Design review of the part shown in the three views and the two pictorial views. Dimensions are in mm from the part's minimum x, y and z. A direction names the side the tool comes from. Give positions to 0.01 mm unless a question says otherwise; leave off trailing zeros. Loops run counter-clockwise (first coordinate to the right, second up) from the corner with the lowest first, then second, coordinate; pieces in that order, holes last. Notation, with made-up numbers: (35.25, 33.5) - (73.25, 33.5) arc R35 ccw to (73.25, 68.5) - close; hole circle Ø10 at (6, 25). An arc over 180 degrees is marked (long way). Answer as a JSON object with one key per item and string values.
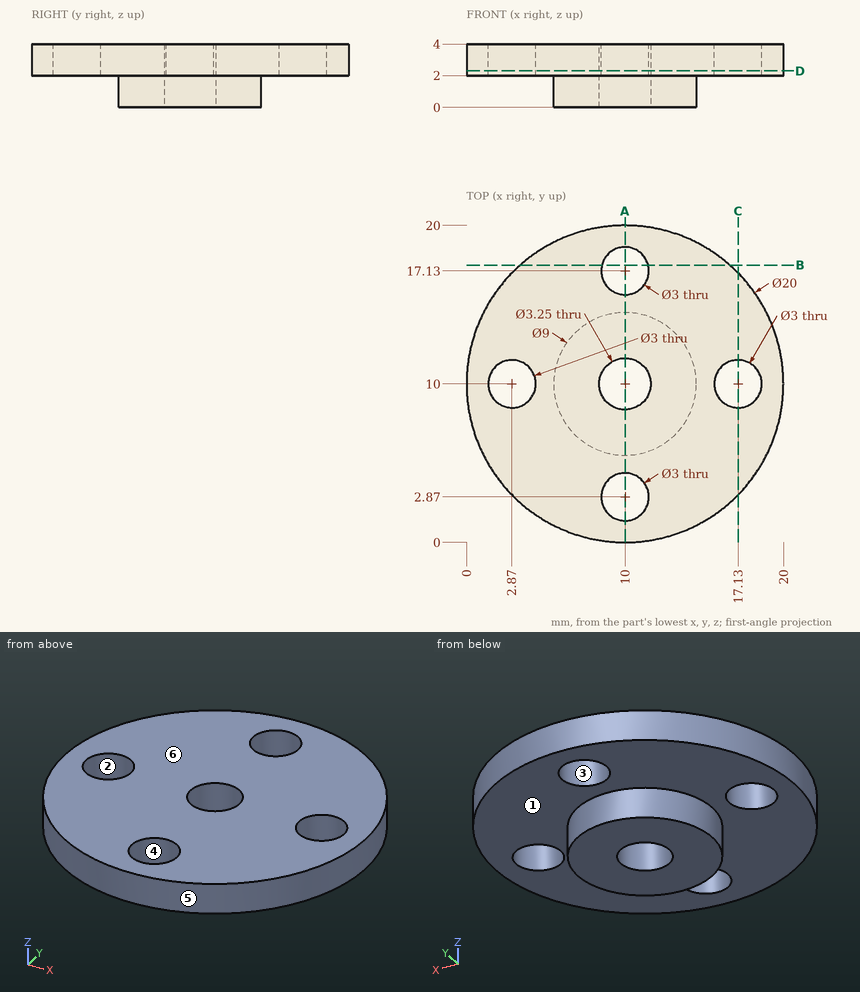
Q1. Clearance check with flat-ended pins moving along their axes: pin 1 Ø4 at (x, y) = (10, 10) entering from +Z; pin 2 Ø3.5 at (x, y) = (10, 2.87) entering from -Z. State where each tip first meets the part, or that it passes through.
Results:
{"pin 1": "stops at z = 4", "pin 2": "stops at z = 2"}
Q2. The part is to be moulded in two halves that separate along X. For the marked faces 3, 4, 5 and 6, say which applies: +X half, -X half, draft (parallel to the pull), parting line (faces both ways), or undercut.
Results:
{"face 3": "undercut", "face 4": "undercut", "face 5": "parting line", "face 6": "draft"}
Q3. Consider section D-D, the plane z = 2.3. State the section outline as (x, y) points (3 decimals).
Results:
{"outline": "circle Ø20 at (10, 10); hole circle Ø3 at (2.87, 10); hole circle Ø3.25 at (10, 10); hole circle Ø3 at (10, 2.87); hole circle Ø3 at (10, 17.13); hole circle Ø3 at (17.13, 10)"}
Q4. For the marked faces 1 and 2, list the 3-axis set-ups (+Z, -Z, +X, -X, +Y, -Y) from which the entire face can be reached by the end or side of a thin tool; tool diameter is ignored.
Results:
{"face 1": "-Z", "face 2": "+Z, -Z"}
Q5. To check wall thickness, follow probe 1 along Y at (x, z) = (10, 3.5) (3 decimals); probe 2 along Y at (x, z) = (9.5, 2.95); probe 3 along Z at (x, y) = (11.75, 18.5). State the ranges of each line that lie inside material, in increasing order. Write a range as [from, to].
Results:
{"probe 1": "y = [0, 1.37], [4.37, 8.375], [11.625, 15.63], [18.63, 20]", "probe 2": "y = [0.01, 1.46], [4.28, 8.45], [11.55, 15.72], [18.54, 19.99]", "probe 3": "z = [2, 4]"}
Q6. Consider section C-C, the plane x = 17.13. State the section outline as (y, z) points, plus the area to 3 significant figures.
Results:
{"outline": "(2.99, 2) - (8.5, 2) - (8.5, 4) - (2.99, 4) - close; (11.5, 2) - (17.01, 2) - (17.01, 4) - (11.5, 4) - close", "area": "22.0 mm^2"}
Q7. Consider section A-A, the plane x = 10. State the section outline as (y, z) points (3 decimals), plus the area to 3 significant figures.
Results:
{"outline": "(0, 2) - (1.37, 2) - (1.37, 4) - (0, 4) - close; (4.37, 2) - (5.5, 2) - (5.5, 0) - (8.375, 0) - (8.375, 4) - (4.37, 4) - close; (11.625, 0) - (14.5, 0) - (14.5, 2) - (15.63, 2) - (15.63, 4) - (11.625, 4) - close; (18.63, 2) - (20, 2) - (20, 4) - (18.63, 4) - close", "area": "33.0 mm^2"}
Q8. Consider section B-B, the plane y = 17.5. State the section outline as (x, z) points, plus the area to 3 significant figures.
Results:
{"outline": "(3.39, 2) - (8.55, 2) - (8.55, 4) - (3.39, 4) - close; (11.45, 2) - (16.61, 2) - (16.61, 4) - (11.45, 4) - close", "area": "20.6 mm^2"}
